Design review of the part built by this model. Coordinates are the model's own, in mm. Face numbers are marked on the shaded views. Coordinates: 2 decimals unless noted, no trailing zeros. Order: outer loops, then holes, each group sorted by start corner. A loop starts at its lowest first (then second) coordinate and runs counter-clockwise, first axis right, second up.
Autodesk Inventor part; units mm, degrees
ref_plane "YZ Plane" through (0, 0, 0) normal (1, 0, 0) x (0, 1, 0)
ref_plane "XZ Plane" through (0, 0, 0) normal (0, 1, 0) x (-1, 0, 0)
ref_plane "XY Plane" through (0, 0, 0) normal (0, 0, 1) x (1, 0, 0)
sketch "Sketch3" plane through (0, 0, 0) normal (1, 0, 0) x (0, 1, 0)
  line L0 (0, 0) -> (0, -35)
  line L1 (-17.5736, -77.4264) -> (-42.3223, -102.1751)
  arc A0 (-17.5736, -77.4264) -> (0, -35) centre (-60, -35) ccw
  point P0 (0, -59.8528)
  point P1 (0, -15)
  point P2 (-31.8934, -91.7462)
  dimension "d36" = 135
  dimension "d37" = 60
  dimension "d41" = 15
  dimension "d50" = 35
sketch "Sketch1" plane through (0, 0, 0) normal (0, 0, 1) x (1, 0, 0)
  circle A0 centre (0, 0) radius 22
  circle A1 centre (0, 0) radius 26.5
  dimension "d1" = 53
  dimension "d2" = 44
sweep "Sweep1" add profiles "Sketch1" path "Sketch3"
hole "Hole3" at (0, 0, -15) at (0, -31.8934, -91.7462) direction (-1, 0, 0) diameter 8.376 end through all
fillet "Fillet3" radius 2 2 edges at (-26.5, 0, 0) (-26.5, -42.3223, -102.1751)
properties part number "55-7" material "Iron, Cast"
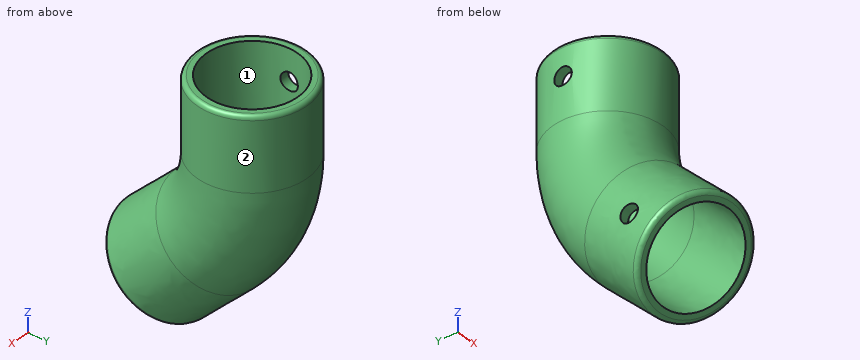
1. Add section A-A (z = -26). Give the boundary of the cut face in (x, y).
2. To check wall thickness, follow line 1 (Y direction, x = 0, z = -25.5); line 2 (X direction, y = 0, z = -11); line 3 (X direction, y = -20, z = -28.5). State the ranges of each line that lie inside material, in increasing order.
3. Insertion check: pin 1 (4 mm diameter, centred on x = 1.5, y = -33.5, fed in from +Z); pin 2 (6 mm diameter, centred on x = 17, z = -46, fed in from -Y); pin 3 (10 mm diameter, centred on x = -20, z = -34, fed in from -Y). Each pin has a flat end and moves straight along its axis. Give the tip position at first contact, or say it passes through.
4. Mouldability with a two-part tool opening along Y and no side actions: class the marked faces 1 and 2 as pulls with the +Y half, pulls with the -Y half, needs draft (parallel to the pull), parting line crosses it, or undercut.
Solution:
1. outline: circle Ø53 at (0, 0); hole circle Ø44 at (0, 0)
2. line 1: y = -26.5 to -22, 22 to 26.5
2. line 2: x = 22 to 26.5
2. line 3: x = -17.39 to -9.17, 9.17 to 17.39
3. pin 1: stops at z = -52.68
3. pin 2: stops at y = -24.38
3. pin 3: stops at y = -21.85
4. face 1: undercut
4. face 2: parting line crosses it
